Autodesk Inventor part; units mm, degrees
ref_plane "YZ Plane" through (0, 0, 0) normal (1, 0, 0) x (0, 1, 0)
ref_plane "XZ Plane" through (0, 0, 0) normal (0, 1, 0) x (-1, 0, 0)
ref_plane "XY Plane" through (0, 0, 0) normal (0, 0, 1) x (1, 0, 0)
sketch "Sketch1" plane through (0, 0, 0) normal (0, 1, 0) x (-1, 0, 0)
  circle A0 centre (0, 0) radius 50
  dimension "d0" = 100
extrude "Extrusion1" add sketch "Sketch1" along normal blind 2
sketch "Sketch2" plane through (0, 2, 0) normal (0, 1, 0) x (1, 0, 0)
  circle A0 centre (0, 0) radius 50
  circle A1 centre (0, 0) radius 45
  dimension "d3" = 5
extrude "Extrusion2" add sketch "Sketch2" along normal blind 3
fillet "Fillet1" radius 2 2 edges at (-45, 5, 0) (-50, 5, 0)
sketch "Sketch3" plane through (0, 0, 0) normal (0, 0, 1) x (1, 0, 0)
  line L0 (-50, 0) -> (50, 0)
  line L1 (0, 0) -> (-13, 0)
  line L2 (-13, 0) -> (13, 0)
  line L3 (13, 0) -> (13, 2)
  line L4 (13, 2) -> (-13, 2)
  line L5 (-13, 2) -> (-13, 0)
  dimension "d7" = 13
  dimension "d8" = 26
  dimension "d9" = 2
extrude "Extrusion3" cut sketch "Sketch3" against normal through all
equation "\"d7\" = 0.5 * d8"
properties part number "mug_base"
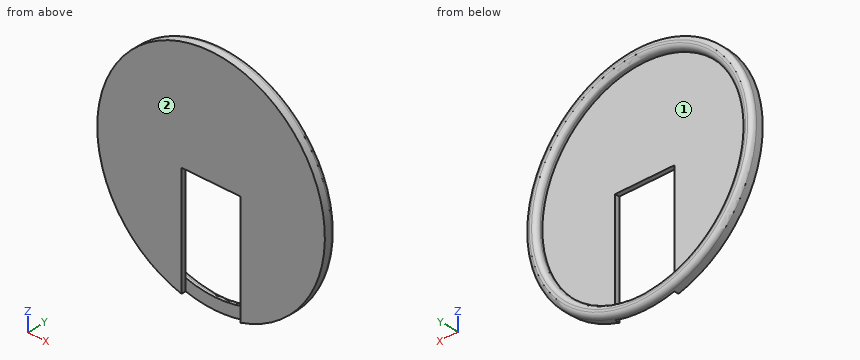
Check sheet for the modelled part. Datum: model origin and axes. Units: mm. Face numbers are marked on the shaded views. Round coordinates to 2 decimals unless told otherwise and drop trailing zeros. Loops run counter-clockwise (first coordinate to the right, second up) from the corner with the lowest first, then second, coordinate; pieces in that order, holes last. Notation, with made-up numbers: (-15.75, -8.75) -> (39.25, -8.75) arc R26 cw to (39.25, 22.25) -> close; hole circle Ø7 at (-38.5, 36). An arc over 180 degrees is marked (long way). Write item = value, one per line. Start each with the question number.
1) Release check for a two-part mould opening along X. For the marked faces 1 and 2 record: released by +X, released by -X, zero draft, split by the parting line, or undercut.
2) Gauge pin test, flat ends, axial feed: pin 1 Ø3 at (y, z) = (3.5, 33) entering from +X; pin 2 Ø1 at (x, y) = (28, 1) entering from +Z; pin 3 Ø2 at (y, z) = (1, -22) entering from +X. Record the tip position at first contact, or that the pin passes through.
3) Sectioned sample at B-B, the plane y = 1.05. Record the cut outline in (x, z), plus the area to 3 significant figures.
4) Thickness scan on probe 1 along Z at (x, y) = (0, 2.55); probe 2 along Y at (x, z) = (-11, 43). Record the ranges inside material, lowest first.
Results are:
q1.face_1 = undercut
q1.face_2 = zero draft
q2.pin_1 = 38.79
q2.pin_2 = 41.76
q2.pin_3 = 45.38
q3.outline = (-13, -48.28) -> (-13, 0) -> (13, 0) -> (13, -48.28) arc R50 ccw (long way) to start
q3.area = 6,570 mm^2
q4.probe_1 = -50 to -45, 45 to 50
q4.probe_2 = 0 to 2
